Autodesk Inventor part; units mm, degrees
ref_plane "YZ Plane" through (0, 0, 0) normal (1, 0, 0) x (0, 1, 0)
ref_plane "XZ Plane" through (0, 0, 0) normal (0, 1, 0) x (-1, 0, 0)
ref_plane "XY Plane" through (0, 0, 0) normal (0, 0, 1) x (1, 0, 0)
sketch "Sketch1" plane through (0, 0, 0) normal (0, 0, 1) x (1, 0, 0)
  circle A0 centre (0, 0) radius 3.625
  dimension "d0" = 7.25
extrude "Extrusion1" add sketch "Sketch1" along normal blind 22
sketch "Sketch2" plane through (0, 0, 0) normal (0, 0, -1) x (-1, 0, 0)
  arc A0 (4.6, 4.3046) -> (-6.3, 0) centre (0, 0) ccw
  line L0 (4.6, 4.3046) -> (4.6, -9.8)
  line L1 (-6.3, 0) -> (-6.3, -9.8)
  line L2 (-6.3, -9.8) -> (4.6, -9.8)
  dimension "d3" = 6.3
  dimension "d4" = 4.6
  dimension "d5" = 9.8
extrude "Extrusion2" add sketch "Sketch2" against normal blind 1.25
sketch "Sketch3" plane through (0, 0, 0) normal (0, 0, -1) x (-1, 0, 0)
  circle A0 centre (0, 0) radius 2.2
  dimension "d8" = 4.4
extrude "Extrusion3" cut sketch "Sketch3" against normal blind 16
sketch "Sketch4" plane through (0, 0, 22) normal (0, 0, 1) x (1, 0, 0)
  circle A0 centre (0, 0) radius 2.2
  circle A1 centre (0, 0) radius 1.25
  dimension "d11" = 2.5
extrude "Extrusion4" cut sketch "Sketch4" against normal up to next contours A1
chamfer "Chamfer1" distance 1.4 angle 45 1 edges at (2.2, 0, 0)
sketch "Sketch5" plane through (0, 0, 0) normal (0, 1, 0) x (-1, 0, 0)
  line L0 (3.625, 1.25) -> (3.625, 22)
  line L1 (-3.625, 1.25) -> (-3.625, 22)
  line L2 (3.625, 22) -> (-3.625, 22)
  line L3 (3.625, 17) -> (1.8, 17)
  line L4 (1.8, 17) -> (1.8, 22)
  line L5 (1.8, 22) -> (3.625, 22)
  line L6 (3.625, 22) -> (3.625, 17)
  line L7 (-3.6, 0) -> (3.6, 0)
  line L8 (1.8, 17) -> (3.625, 15.9463)
  line L9 (3.625, 1.25) -> (3.625, 22)
  line L10 (1.8, 17) -> (3.9073, 17) construction
  line L11 (3.625, 15.9463) -> (3.625, 17)
  point P0 (0, 0)
  dimension "d17" = 5.425
  dimension "d18" = 17
  dimension "d21" = 30
extrude "Extrusion5" cut sketch "Sketch5" along normal through all both and the other way through all
sketch "Sketch6" plane through (0, 0, 0) normal (0, 1, 0) x (-1, 0, 0)
  line L0 (1.8, 22) -> (-3.625, 22)
  line L1 (-1.25, 22) -> (1.25, 22)
  line L2 (0, 22) -> (0, 19.2621) construction
  circle A0 centre (-4.6, 23.4) radius 4.6
  circle A1 centre (5.4, 23.4) radius 5.4
  line L3 (12.1762, 23.4) -> (-11.9471, 23.4)
  point P0 (0, 0)
  dimension "d22" = 4.6
  dimension "d23" = 5.4
  dimension "d24" = 1.4
extrude "Extrusion6" cut sketch "Sketch6" along normal through all both and the other way through all contours A1 L3 | A0 L3 | L3 A0 | A1 L3
sketch "Sketch7" plane through (0, 0, 0) normal (1, 0, 0) x (0, 1, 0)
  line L0 (-3.1465, 19.3751) -> (3.1465, 19.3751)
  line L1 (1.2308, 22) -> (3.6184, 22)
  line L2 (3.6184, 22) -> (3.6184, 24.6476)
  line L3 (0, 19.6751) -> (0, 24.6476) construction
  circle A0 centre (0, 23.2935) radius 3.6184
  point P0 (0, 0)
  point P1 (0, 19.3751)
  dimension "d29" = 0.3
extrude "Extrusion7" cut sketch "Sketch7" along normal through all both and the other way through all contours A0
properties part number "guide tube"
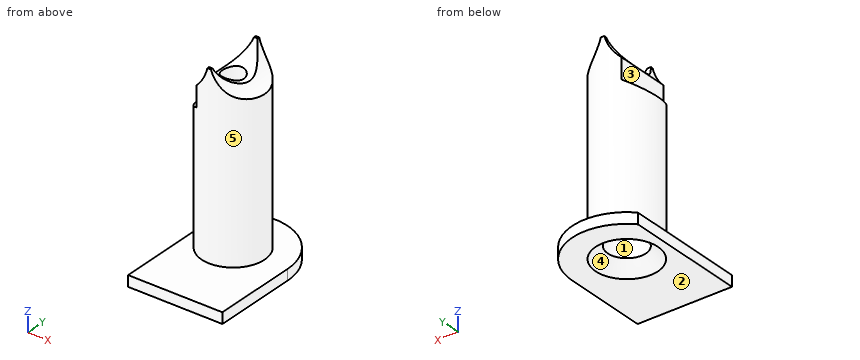
The listing builds one solid part. Answer for the finished solid, in the listing's coordinates (mm). Face numbers are marked on the shaded views. A direction names the side the tool comes from. Coordinates: 2 decimals unless noted, no trailing zeros. Write each loop counter-clockwise with the first axis right and the second up, starting at its lowest first coordinate (ties: lowest second). Pieces come first, ordered by that corner, then holes. Notation, with made-up numbers: M -27,57 L 22,57 A21 cw 22,75 Z; hole C 18,-9 d11. An arc over 180 degrees is marked long. Use one line per item in the form item = value.
Item 1: Find section A-A, the plane z = 2.5. Give the vertices of the cut face in (x, y) (3 decimals), plus the area to 3 significant figures.
Model answer:
outline = C 0,0 d7.25; hole C 0,0 d4.4
area = 26.1 mm2
Item 2: Find section B-B, the plane x = 4.25. Give the vertices of the cut face in (y, z).
Model answer:
outline = M -9.8,0 L 4.65,0 L 4.65,1.25 L -9.8,1.25 Z
Item 3: For the marked faces 1 and 2, determine the directions among +Z, -Z, +X, -X, +Y, -Y from which every point of the face is accessible in a straight line to the end or side of a thin tool.
Model answer:
face_1 = -Z
face_2 = -Z, +X, -X, +Y, -Y
Item 4: The mould has two halves that part along Y. Classify the marked faces 3, 4 and 5: released by +Y, released by -Y, zero draft, split by the parting line, or undercut.
Model answer:
face_3 = zero draft
face_4 = undercut
face_5 = split by the parting line
Item 5: Find the intervals of material crossed by probe 1 along X at (y, z) = (0, 17.5) (3 decimals); probe 2 along Y at (x, z) = (0, 17.25) (3 decimals); probe 3 along Y at (x, z) = (0, 7.25) (3 decimals), in increasing order.
Model answer:
probe_1 = -1.8 to -1.25, 1.25 to 3.625
probe_2 = -3.625 to -1.25, 1.25 to 3.625
probe_3 = -3.625 to -2.2, 2.2 to 3.625
Item 6: Given P1, Ø4, axis at x = 0, y = 0, coming from the +Z side; P2, Ø1.5, axis at y = 4, z = 2.5, coming from the +X side; P3, Ø1.5, axis at y = -1.5, z = 13.5, coming from the +X side; P4, Ø2, axis at x = 0, y = 0, coming from the -Z side, each flat-ended and moving along its own axis, determine where each tip first touches the part or whether it passes through.
Model answer:
P1 = 20.28
P2 = 1.61
P3 = 3.55
P4 = through
